Geometry: final body of the model. Coordinates: model frame, mm. Face numbers are marked on the shaded views. A direction names the side the tool comes from. Coordinates: 2 decimals unless noted, no trailing zeros. Use CSV: the item, a comma, the result in double quotes. Start each with the question number.
Q1. Ray query, probe 1 along Y at (x, z) = (-1.5, 4.5); probe 2 along Z at (x, y) = (16.5, 33); probe 3 along Z at (x, y) = (-18, -13). Return the intervals inside material, ascending.
Q2. Access query for the marked faces 1, 2 and 3. Directions: +Z, -Z, +X, -X, +Y, -Y. A direction counts if a zero-diameter tool reaches every point of the face in a straight line with its end or side. Return the directions, or none.
Q3. Mould query, pull axis Y, two halves, no side actions, for the marked faces 4, 5 and 6. Classes: +Y half, -Y half, draft (parallel to the pull), parting line (faces both ways), or undercut.
Q4. First-contact query: P1, Ø8, axis at y = 1, z = -4.5, coming from the -X side; P2, Ø6, axis at y = 37, z = 4.5, coming from the +X side; P3, Ø10, axis at x = -31, z = 6, coming from the +Y side; P4, Ø16, axis at x = 10, y = -4.5, coming from the -Z side. Flat tips, straight axial feed; report the tip coordinate or a pass-through.
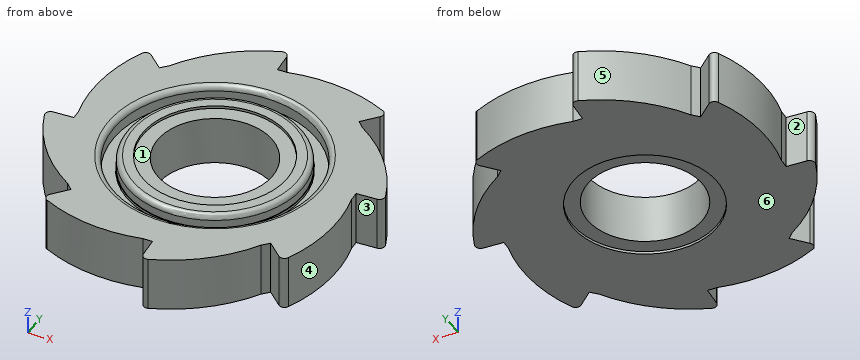
from build123d import *

# Parameters (mm, degrees)
SKETCH1_R           = 21
BOSS_EXTRUDE1_DEPTH = 10
SKETCH11_R          = 26.424144251
CUT_EXTRUDE2_DEPTH  = 1
FILLET1_R           = 2
SKETCH12_R          = 37
SKETCH12_R_2        = 32.216977435
CUT_EXTRUDE3_DEPTH  = 5
SKETCH13_R          = 37
SKETCH13_R_2        = 32
CUT_EXTRUDE5_DEPTH  = 5
FILLET2_R           = 2


with BuildPart() as part:
    # Sketch1 → Boss-Extrude1 (new body)
    with BuildSketch(Plane.XY):
        with BuildLine():
            Line((49.887269323, 3.355645919), (59.864723187, 4.026775102))
            ThreePointArc((59.864723187, 4.026775102), (50.436634414, 21.90240344), (35.355339059, 35.355339059))
            ThreePointArc((35.355339059, 35.355339059), (34.148336007, 36.52247456), (32.902826449, 37.648426417))
            Line((32.902826449, 37.648426417), (39.483391738, 45.178111701))
            ThreePointArc((39.483391738, 45.178111701), (20.176748218, 51.151424211), (0, 50))
            ThreePointArc((0, 50), (-1.67876947, 49.971809384), (-3.355645919, 49.887269323))
            Line((-3.355645919, 49.887269323), (-4.026775102, 59.864723187))
            ThreePointArc((-4.026775102, 59.864723187), (-21.90240344, 50.436634414), (-35.355339059, 35.355339059))
            ThreePointArc((-35.355339059, 35.355339059), (-36.52247456, 34.148336007), (-37.648426417, 32.902826449))
            Line((-37.648426417, 32.902826449), (-45.178111701, 39.483391738))
            ThreePointArc((-45.178111701, 39.483391738), (-51.151424211, 20.176748218), (-50, 0))
            ThreePointArc((-50, 0), (-49.971809384, -1.67876947), (-49.887269323, -3.355645919))
            Line((-49.887269323, -3.355645919), (-59.864723187, -4.026775102))
            ThreePointArc((-59.864723187, -4.026775102), (-50.436634414, -21.90240344), (-35.355339059, -35.355339059))
            ThreePointArc((-35.355339059, -35.355339059), (-34.148336007, -36.52247456), (-32.902826449, -37.648426417))
            Line((-32.902826449, -37.648426417), (-39.483391738, -45.178111701))
            ThreePointArc((-39.483391738, -45.178111701), (-20.176748218, -51.151424211), (0, -50))
            ThreePointArc((0, -50), (1.67876947, -49.971809384), (3.355645919, -49.887269323))
            Line((3.355645919, -49.887269323), (4.026775102, -59.864723187))
            ThreePointArc((4.026775102, -59.864723187), (21.90240344, -50.436634414), (35.355339059, -35.355339059))
            ThreePointArc((35.355339059, -35.355339059), (36.52247456, -34.148336007), (37.648426417, -32.902826449))
            Line((37.648426417, -32.902826449), (45.178111701, -39.483391738))
            ThreePointArc((45.178111701, -39.483391738), (51.151424211, -20.176748218), (50, 0))
            ThreePointArc((50, 0), (49.971809384, 1.67876947), (49.887269323, 3.355645919))
        make_face()
        Circle(SKETCH1_R, mode=Mode.SUBTRACT)
    boss_extrude1 = extrude(amount=BOSS_EXTRUDE1_DEPTH)

    # Sketch11 → Cut-Extrude2 (cut)
    with BuildSketch(Plane.XY.offset(10)):
        Circle(SKETCH11_R)
    cut_extrude2 = extrude(amount=-CUT_EXTRUDE2_DEPTH, mode=Mode.SUBTRACT)

    # Mirror1: Boss-Extrude1, Cut-Extrude2 across Front Plane
    add(boss_extrude1.mirror(Plane.XY))
    add(cut_extrude2.mirror(Plane.XY), mode=Mode.SUBTRACT)

    # Fillet1
    fillet1_edges = [part.edges().sort_by_distance(p)[0] for p in [
        (59.864723187, 4.026775102, 0),
        (45.178111701, -39.483391738, 0),
        (4.026775102, -59.864723187, 0),
        (-39.483391738, -45.178111701, 0),
        (-59.864723187, -4.026775102, 0),
        (-45.178111701, 39.483391738, 0),
        (-4.026775102, 59.864723187, 0),
        (39.483391738, 45.178111701, 0),
    ]]
    fillet(fillet1_edges, radius=FILLET1_R)

    # Sketch12 → Cut-Extrude3 (cut)
    with BuildSketch(Plane.XY.offset(9)):
        Circle(SKETCH12_R)
        Circle(SKETCH12_R_2, mode=Mode.SUBTRACT)
    extrude(amount=-CUT_EXTRUDE3_DEPTH, mode=Mode.SUBTRACT)

    # Sketch13 → Cut-Extrude5 (cut)
    with BuildSketch(Plane.XY.offset(10)):
        Circle(SKETCH13_R)
        Circle(SKETCH13_R_2, mode=Mode.SUBTRACT)
    extrude(amount=-CUT_EXTRUDE5_DEPTH, mode=Mode.SUBTRACT)

    # Fillet2
    fillet2_edges = [part.edges().sort_by_distance(p)[0] for p in [
        (-37, 0, 10),
        (-32, 0, 10),
    ]]
    fillet(fillet2_edges, radius=FILLET2_R)


solid = part.part
Responses:
1,probe 1,"y = -50.34 to -36.97, -32.18 to -20.95, 20.95 to 32.18, 36.97 to 49.98"
1,probe 2,"z = -10 to 4"
1,probe 3,"z = -9 to 9"
2,face 1,"+Z"
2,face 2,"+Z, -Z, -X"
2,face 3,"+Z, -Z, +X"
3,face 4,"undercut"
3,face 5,"+Y half"
3,face 6,"draft"
4,P1,"stops at x = -50.97"
4,P2,"stops at x = 37.46"
4,P3,"stops at y = 46.9"
4,P4,"passes through"
